Check sheet for the drawn part. Datum: minimum x, y, z corner. Units: mm. A direction names the side the tool comes from. Round coordinates to 2 decimals unless told otherwise and drop trailing zeros. Write each loop counter-clockwise with the first axis right and the second up, starting at its lowest first coordinate (ties: lowest second). Pieces come first, ordered by that corner, then holes. Notation, with made-up numbers: (68, -0.75) - (118, -0.75) arc R9 cw to (118, 16.25) - close; hole circle Ø1 at (14.25, 2). An arc over 180 degrees is marked (long way). Answer as a JSON object with one key per item and string values. Group by question number.
1) Section check B-B (x = 9.95). Enter the section's corners in (y, z), then the cut area to 3 significant figures.
2) Set-up check for the marked faces 1 and 2: record each of +Z, -Z, +X, -X, +Y, -Y from which the full face is reachable in a straight line by a thin tool's end or side.
3) Go/stop test with flat-tipped pins: pin 1 Ø4 at (y, z) = (20.5, 68) entering from +X; pin 2 Ø6 at (y, z) = (15.5, 57.5) entering from +X; pin 3 Ø8 at (y, z) = (27, 18.5) entering from +X; pin 4 Ø1.5 at (y, z) = (10.5, 85) entering from +X. Record where each tip stops, or that it passes through.
4) Section check C-C (x = 64.2). Enter the section's corners in (y, z).
5) Section check D-D (z = 33.5). Enter the section's corners in (x, y).
6) Section check A-A (z = 64.2). State how many separate pieces and enclosed holes the cut face has, then the cut area to 3 significant figures.
7) Thickness scan on line 1 (X direction, y = 47, z = 64); line 2 (Y direction, x = 101, z = 54); line 3 (Y direction, x = 27, z = 113). Record the ranges inside material, lowest first.
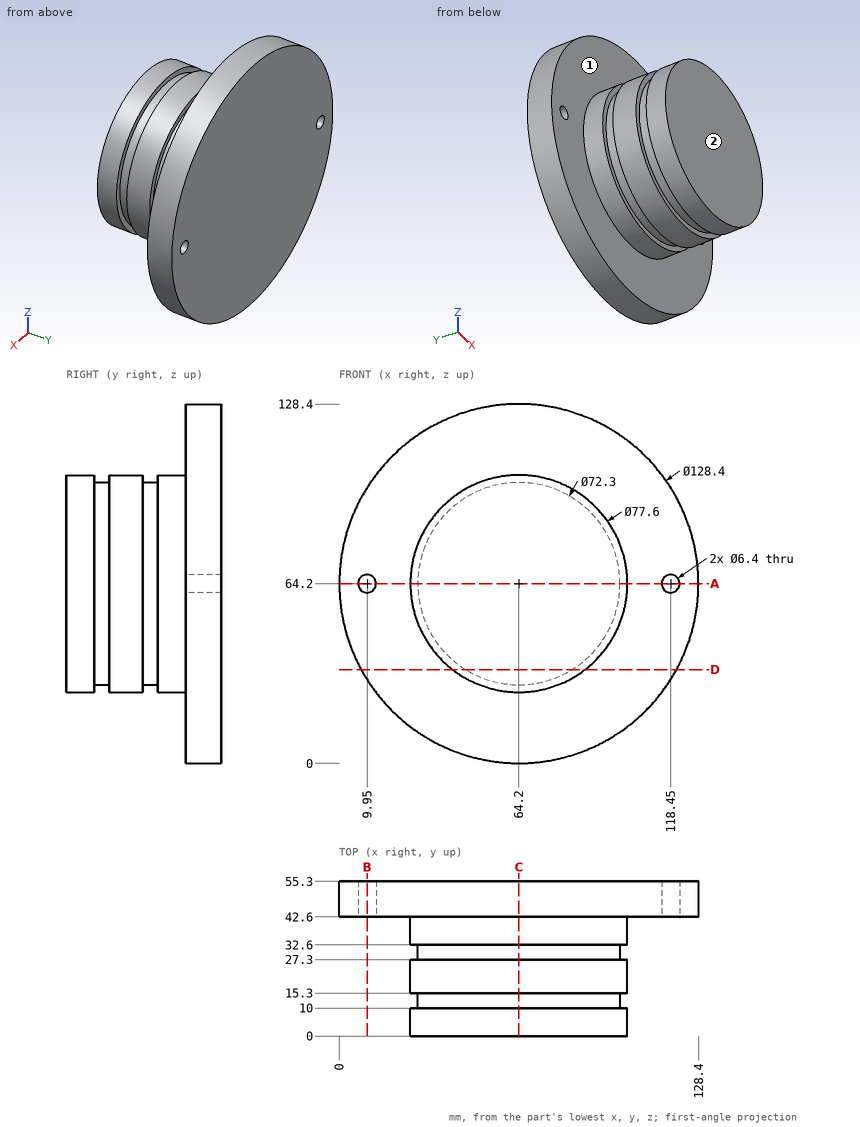
Returned:
{
 "1": {"outline": "(42.6, 29.87) - (55.3, 29.87) - (55.3, 61) - (42.6, 61) - close; (42.6, 67.4) - (55.3, 67.4) - (55.3, 98.53) - (42.6, 98.53) - close", "area": "791 mm2"},
 "2": {"face 1": "-Y", "face 2": "+Z, -Z, +X, -X, -Y"},
 "3": {"pin 1": "x = 102.96", "pin 2": "x = 102.82", "pin 3": "through", "pin 4": "x = 97.3"},
 "4": {"outline": "(0, 25.4) - (10, 25.4) - (10, 28.05) - (15.3, 28.05) - (15.3, 25.4) - (27.3, 25.4) - (27.3, 28.05) - (32.6, 28.05) - (32.6, 25.4) - (42.6, 25.4) - (42.6, 0) - (55.3, 0) - (55.3, 128.4) - (42.6, 128.4) - (42.6, 103) - (32.6, 103) - (32.6, 100.35) - (27.3, 100.35) - (27.3, 103) - (15.3, 103) - (15.3, 100.35) - (10, 100.35) - (10, 103) - (0, 103) - close"},
 "5": {"outline": "(7.82, 42.6) - (40.47, 42.6) - (40.47, 32.6) - (45.11, 32.6) - (45.11, 27.3) - (40.47, 27.3) - (40.47, 15.3) - (45.11, 15.3) - (45.11, 10) - (40.47, 10) - (40.47, 0) - (87.93, 0) - (87.93, 10) - (83.29, 10) - (83.29, 15.3) - (87.93, 15.3) - (87.93, 27.3) - (83.29, 27.3) - (83.29, 32.6) - (87.93, 32.6) - (87.93, 42.6) - (120.58, 42.6) - (120.58, 55.3) - (7.82, 55.3) - close"},
 "6": {"separate pieces": "3", "enclosed holes": "0", "area": "4,720 mm2"},
 "7": {"line 1": "0 to 6.76, 13.14 to 115.26, 121.64 to 128.4", "line 2": "0 to 10, 15.3 to 27.3, 32.6 to 55.3", "line 3": "42.6 to 55.3"}
}
